Verification items for the finished model (mm, model axes). A direction names the side the tool comes from. Round coordinates to 2 decimals unless told otherwise and drop trailing zeros. Write each loop counter-clockwise with the first axis right and the second up, starting at its lowest first coordinate (ties: lowest second). Pieces come first, ordered by that corner, then holes. Notation, with made-up numbers: M 38.5,83.5 L 69.5,83.5 A23 ccw 69.5,100.5 Z; hole C 1.5,-7.5 d5. An arc over 180 degrees is marked long. One line per item, written item: value. Start each with the question number.
Autodesk Inventor part; units mm, degrees
ref_plane "YZ Plane" through (0, 0, 0) normal (1, 0, 0) x (0, 1, 0)
ref_plane "XZ Plane" through (0, 0, 0) normal (0, 1, 0) x (-1, 0, 0)
ref_plane "XY Plane" through (0, 0, 0) normal (0, 0, 1) x (1, 0, 0)
sketch "Sketch1" plane through (0, 0, 0) normal (0, 0, 1) x (1, 0, 0)
  line L0 (0, 0) -> (72.4, 0)
  line L1 (72.4, 0) -> (72.4, 71)
  line L2 (72.4, 71) -> (0, 71)
  line L3 (0, 71) -> (0, 0)
  dimension "d0" = 72.4
  dimension "d1" = 71
extrude "Extrusion1" add sketch "Sketch1" along normal blind 10
sketch "Sketch2" plane through (0, 0, 10) normal (0, 0, 1) x (1, 0, 0)
  line L0 (72.4, 71) -> (0, 71)
  line L1 (52.4, 71) -> (12.4, 71)
  line L2 (12.4, 71) -> (12.4, 81)
  line L3 (12.4, 81) -> (52.4, 81)
  line L4 (52.4, 81) -> (52.4, 71)
  circle A0 centre (32.4, 76) radius 2.5
  line L5 (72.4, 0) -> (72.4, 71)
  point P0 (0, 0)
  point P1 (52.4, 76)
  point P2 (32.4, 81)
  dimension "d4" = 40
  dimension "d5" = 10
  dimension "d6" = 5
  dimension "d7" = 20
extrude "Extrusion2" add sketch "Sketch2" against normal blind 5
sketch "Sketch3" plane through (0, 0, 10) normal (0, 0, 1) x (1, 0, 0)
  line L0 (0, 71) -> (0, 0)
  line L1 (0, 0) -> (-19, 0)
  line L2 (-19, 0) -> (-19, 71)
  line L3 (-19, 71) -> (0, 71)
  line L4 (0, 71) -> (0, 0)
  line L5 (12.4, 71) -> (0, 71)
  circle A0 centre (-9.5, 35.5) radius 2.5
  point P0 (-19, 35.5)
  point P1 (-9.5, 71)
  dimension "d10" = 19
  dimension "d13" = 5
extrude "Extrusion3" add sketch "Sketch3" against normal blind 10
sketch "Sketch4" plane through (0, 0, 10) normal (0, 0, 1) x (1, 0, 0)
  line L0 (-19, 0) -> (72.4, 0)
  line L1 (52.4, 0) -> (12.4, 0)
  line L2 (12.4, 0) -> (12.4, 10)
  line L3 (12.4, 10) -> (52.4, 10)
  line L4 (52.4, 10) -> (52.4, 0)
  line L5 (72.4, 0) -> (72.4, 71)
  line L6 (72.4, 55.5) -> (62.4, 55.5)
  line L7 (62.4, 55.5) -> (62.4, 15.5)
  line L8 (62.4, 15.5) -> (72.4, 15.5)
  line L9 (72.4, 15.5) -> (72.4, 55.5)
  point P0 (0, 0)
  point P1 (72.4, 35.5)
  point P2 (72.4, 35.5)
  point P3 (52.4, 81)
  dimension "d16" = 40
  dimension "d17" = 10
  dimension "d18" = 10
  dimension "d19" = 40
extrude "Extrusion4" cut sketch "Sketch4" against normal blind 5 contours L8 L7 L6 L5
sketch "Sketch5" plane through (0, 0, 5) normal (0, 0, 1) x (1, 0, 0)
  line L0 (62.4, 55.5) -> (72.4, 55.5) construction
  line L1 (62.4, 15.5) -> (62.4, 55.5) construction
  line L2 (72.4, 15.5) -> (62.4, 15.5) construction
  line L3 (72.4, 55.5) -> (72.4, 15.5) construction
  line L4 (52.4, 10) -> (52.4, 0) construction
  line L5 (12.4, 10) -> (52.4, 10) construction
  line L6 (12.4, 0) -> (12.4, 10) construction
  line L7 (52.4, 0) -> (12.4, 0) construction
  circle A0 centre (32.4, 5) radius 2.5
  circle A1 centre (67.4, 35.5) radius 2.5
  point P0 (0, 0)
  point P1 (62.4, 35.5)
  point P2 (12.4, 5)
  point P3 (67.4, 55.5)
  point P4 (32.4, 10)
  dimension "d22" = 5
  dimension "d23" = 5
extrude "Extrusion5" cut sketch "Sketch5" against normal through all contours A1
properties part number "SP005" material "ABS Plastic"
1) Gauge pin test, flat ends, axial feed: pin 1 Ø4 at (y, z) = (76.5, 7) entering from -X; pin 2 Ø4 at (x, y) = (32.4, 76) entering from -Z; pin 3 Ø2.5 at (y, z) = (32, 8) entering from +X; pin 4 Ø11 at (x, y) = (33.5, 77.5) entering from -Z. Record the tip position at first contact, or that the pin passes through.
2) Mould release check, pull along Y, two halves, no side actions. Record for faces 1 (the flat face through (52.4, 76, 8)), 2 (the cylindrical face through (33.55, 73.78, 7.54)), 3 (the flat face through (32, 81, 8)), 4 (the flat face through (67, 55.5, 8)): pulls with the +Y half, pulls with the -Y half, needs draft (parallel to the pull), parting line crosses it, or undercut.
3) Access from +Z, -Z, +X, -X, +Y, -Y to the whole of each face (thin tool, end or side, straight path). Record for faces 5 (the flat face through (32, 73, 5)), 6 (the flat face through (67, 15.5, 8)), 7 (the cylindrical face through (64.9, 35.6, 2.5)), 8 (the flat face through (26, 41, 10)), 9 (the flat face through (12.4, 76, 8)).
4) Cross-section at A-A (x = 32.4). Record the boundary of the cut face in (y, z).
5) Thickness scan on line 1 (Y direction, x = 67.4, z = 2.55); line 2 (Z direction, x = 25, y = 72.5); line 3 (Y direction, x = 32.4, z = 7.7). Record the ranges inside material, lowest first.
6) Cross-section at B-B (y = 35.5). Record the boundary of the cut face in (x, z).
7) Cross-section at D-D (z = 7). Record the boundary of the cut face in (x, y), then the cut area to 3 significant figures.
8) Cross-section at C-C (y = 76). Record the boundary of the cut face in (x, z), then the cut area to 3 significant figures.
Results below:
1. pin 1: stops at x = 12.4
1. pin 2: passes through
1. pin 3: stops at x = 62.4
1. pin 4: stops at z = 5
2. face 1: needs draft
2. face 2: undercut
2. face 3: pulls with the +Y half
2. face 4: undercut
3. face 5: -Z, +X, -X, +Y
3. face 6: +Z, +X
3. face 7: +Z, -Z
3. face 8: +Z, +X, -X, +Y, -Y
3. face 9: +Z, -Z, -X, +Y
4. outline: M 0,0 L 71,0 L 71,5 L 73.5,5 L 73.5,10 L 0,10 Z; M 78.5,5 L 81,5 L 81,10 L 78.5,10 Z
5. line 1: y = 0 to 33, 38 to 71
5. line 2: z = 5 to 10
5. line 3: y = 0 to 73.5, 78.5 to 81
6. outline: M -19,0 L -12,0 L -12,10 L -19,10 Z; M -7,0 L 64.9,0 L 64.9,5 L 62.4,5 L 62.4,10 L -7,10 Z; M 69.9,0 L 72.4,0 L 72.4,5 L 69.9,5 Z
7. outline: M -19,0 L 72.4,0 L 72.4,15.5 L 62.4,15.5 L 62.4,55.5 L 72.4,55.5 L 72.4,71 L 52.4,71 L 52.4,81 L 12.4,81 L 12.4,71 L -19,71 Z; hole C -9.5,35.5 d5; hole C 32.4,76 d5
7. area: 6,450 mm²
8. outline: M 12.4,5 L 29.9,5 L 29.9,10 L 12.4,10 Z; M 34.9,5 L 52.4,5 L 52.4,10 L 34.9,10 Z
8. area: 175 mm²
